Here's how the part is built. I have some questions about the finished solid (model axes, mm). A direction names the side the tool comes from. Round coordinates to 2 decimals unless told otherwise and drop trailing zeros. Write each loop counter-clockwise with the first axis right and the second up, starting at its lowest first coordinate (ties: lowest second). Pieces come first, ordered by that corner, then holes. Notation, with made-up numbers: M 35,42.25 L 85,42.25 A37 ccw 85,78.25 Z; hole C 76.25,-0.5 d2. An arc over 180 degrees is marked long. Use one line per item in the form item = value. Start each with the question number.
Q1. I want a section at C-C on z = 6. List the corners of the cut face in (x, y) for me, and give its area (3 significant figures).
Q2. I want a section at D-D on z = 20.5. List the corners of the cut face in (x, y) for me, and give its area (3 significant figures).
Q3. I want a section at B-B on x = -49.5. List the corners of the cut face in (y, z) for me.
Q4. I'm going to push flat-ended pins straight in: pin 1 Ø0.9 at (x, y) = (-49.5, -2) entering from +Z; pin 2 Ø1.5 at (y, z) = (-1.5, 3.5) entering from +X; pin 3 Ø1.5 at (y, z) = (-1.5, 4) entering from -X. Where does each tip first touch, or does it pass through?
Q5. I need wall thicknesses on line 1 along Z through (x, y) = (-44, -1); line 2 along X through (y, z) = (-1.9, 6.5); line 3 along X through (y, z) = (-2.7, 15). Which ranges of each line are inside material? Lowest first, please. Write a range as from..to.
Q6. I want a section at A-A on y = -1.3. List the corners of the cut face in (x, z) for me, and give its area (3 significant figures).
Q7. For faces 4 (the face through (-28, -1, 20.042)), 5 (the face through (-50, -1, 6.542)), 6 (the face through (-62, -1, 13.042)), which set-ups out of +Z, -Z, +X, -X, +Y, -Y let a thin tool reach every point of the face, with its end or its side?
Q8. We'd pull the mould along X, two halves only. Please class faces 1 (the face through (-18, -1, 23.042)), 2 (the face through (-63.57, -1, 1)), 3 (the face through (-48, -1, 20.042)): +X half, -X half, draft (parallel to the pull), parting line (faces both ways), or undercut.
```python
from build123d import *

# Parameters (mm, degrees)
F0_W     = 2.98
F0_H     = 5
F1_DEPTH = 3


with BuildPart() as f1:
    # F0 (on Front) → F1 (new body)
    with BuildSketch(Plane.XZ):
        with BuildLine():
            Line((-63.569787, -1.958204), (-36.56974, -1.958204))
            ThreePointArc((-36.56974, -1.958204), (-19.584468, 5.495335), (-13.569787, 23.041796))
            Line((-13.569787, 23.041796), (-23.569787, 23.041796))
            Line((-23.569787, 23.041796), (-23.569787, 20.041796))
            Line((-23.569787, 20.041796), (-33.569787, 20.041796))
            Line((-33.569787, 20.041796), (-33.569787, 23.041796))
            Line((-33.569787, 23.041796), (-43.569787, 23.041796))
            Line((-43.569787, 23.041796), (-43.569787, 20.041796))
            Line((-43.569787, 20.041796), (-53.569787, 20.041796))
            Line((-53.569787, 20.041796), (-53.569787, 23.041796))
            Line((-53.569787, 23.041796), (-63.569787, 23.041796))
            Line((-63.569787, 23.041796), (-63.569787, 18.041796))
            Line((-63.569787, 18.041796), (-60.569787, 18.041796))
            Line((-60.569787, 18.041796), (-60.569787, 13.041796))
            Line((-60.569787, 13.041796), (-63.569787, 13.041796))
            Line((-63.569787, 13.041796), (-63.569787, 8.041796))
            Line((-63.569787, 8.041796), (-60.569787, 8.041796))
            Line((-60.569787, 8.041796), (-60.569787, 3.041796))
            Line((-60.569787, 3.041796), (-63.569787, 3.041796))
            Line((-63.569787, 3.041796), (-63.569787, -1.958204))
        make_face()
        with Locations((-50.079787, 4.041796)):
            Rectangle(F0_W, F0_H, mode=Mode.SUBTRACT)
        with Locations((-50.079787, 14.041796)):
            Rectangle(F0_W, F0_H, mode=Mode.SUBTRACT)
    extrude(amount=F1_DEPTH)


solid = f1.part
```
Reported:
q1.outline = M -60.57,-3 L -51.57,-3 L -51.57,0 L -60.57,0 Z; M -48.59,-3 L -19.13,-3 L -19.13,0 L -48.59,0 Z
q1.area = 115 mm^2
q2.outline = M -63.57,-3 L -53.57,-3 L -53.57,0 L -63.57,0 Z; M -43.57,-3 L -33.57,-3 L -33.57,0 L -43.57,0 Z; M -23.57,-3 L -13.5,-3 L -13.5,0 L -23.57,0 Z
q2.area = 90.2 mm^2
q3.outline = M -3,-1.96 L 0,-1.96 L 0,1.54 L -3,1.54 Z; M -3,6.54 L 0,6.54 L 0,11.54 L -3,11.54 Z; M -3,16.54 L 0,16.54 L 0,20.04 L -3,20.04 Z
q4.pin_1 = 20.04
q4.pin_2 = -20.82
q4.pin_3 = -60.57
q5.line_1 = -1.96..20.04
q5.line_2 = -60.57..-51.57, -48.59..-18.71
q5.line_3 = -60.57..-51.57, -48.59..-14.32
q6.outline = M -63.57,-1.96 L -36.57,-1.96 A23.08 ccw -13.57,23.04 L -23.57,23.04 L -23.57,20.04 L -33.57,20.04 L -33.57,23.04 L -43.57,23.04 L -43.57,20.04 L -53.57,20.04 L -53.57,23.04 L -63.57,23.04 L -63.57,18.04 L -60.57,18.04 L -60.57,13.04 L -63.57,13.04 L -63.57,8.04 L -60.57,8.04 L -60.57,3.04 L -63.57,3.04 Z; hole M -51.57,1.54 L -48.59,1.54 L -48.59,6.54 L -51.57,6.54 Z; hole M -51.57,11.54 L -48.59,11.54 L -48.59,16.54 L -51.57,16.54 Z
q6.area = 1,020 mm^2
q7.face_4 = +Z, +Y, -Y
q7.face_5 = +Y, -Y
q7.face_6 = -X, +Y, -Y
q8.face_1 = draft
q8.face_2 = -X half
q8.face_3 = undercut
